Build history of the part. All positions in model axes, mm. A direction names the side the tool comes from. Round coordinates to 2 decimals unless told otherwise and drop trailing zeros. Order: outer loops, then holes, each group sorted by start corner. A loop starts at its lowest first (then second) coordinate and runs counter-clockwise, first axis right, second up. Notation, with made-up numbers: (-31, 24.5) -> (21, 24.5) arc R32 cw to (21, 55.5) -> close; hole circle Ø11 at (68.25, 44). An arc over 180 degrees is marked (long way). Write item = value, one per line.
from build123d import *

# Parameters (mm, degrees)
BOSS_EXTRU_1_DEPTH      = 704
ENL_V_MAT_EXTRU_1_DEPTH = 590
ENL_V_MAT_EXTRU_2_DEPTH = 590
ENL_V_MAT_EXTRU_3_DEPTH = 41
ENL_V_MAT_EXTRU_4_DEPTH = 41


with BuildPart() as part:
    # Esquisse1 → Boss.-Extru.1 (new body)
    with BuildSketch(Plane(origin=(0, 0, 0), x_dir=(1, 0, 0), z_dir=(0, 1, 0))):
        Polygon((-20, 20.113636364), (20, 20.113636364), (20, 18.113636364), (-18, 18.113636364), (-18, -19.886363636), (-20, -19.886363636), align=None)
    extrude(amount=BOSS_EXTRU_1_DEPTH)

    # Esquisse2 → Enlèv. mat.-Extru.1 (cut)
    with BuildSketch(Plane(origin=(0, 0, -20.113636364), x_dir=(-1, 0, 0), z_dir=(0, 0, -1))):
        Polygon((20, 0), (-20, 40), (-20, 0), align=None)
    extrude(amount=-ENL_V_MAT_EXTRU_1_DEPTH, mode=Mode.SUBTRACT)

    # Esquisse3 → Enlèv. mat.-Extru.2 (cut)
    with BuildSketch(Plane.ZY.offset(20)):
        Polygon((-20.113636364, 0), (19.886363636, 40), (19.886363636, 0), align=None)
    extrude(amount=-ENL_V_MAT_EXTRU_2_DEPTH, mode=Mode.SUBTRACT)

    # Esquisse4 → Enlèv. mat.-Extru.3 (cut, through all)
    with BuildSketch(Plane.ZY.offset(20)):
        Polygon((-20.113636364, 704), (19.886363636, 664), (19.886363636, 704), align=None)
    extrude(amount=-ENL_V_MAT_EXTRU_3_DEPTH, mode=Mode.SUBTRACT)

    # Esquisse5 → Enlèv. mat.-Extru.4 (cut, through all)
    with BuildSketch(Plane(origin=(0, 0, -20.113636364), x_dir=(-1, 0, 0), z_dir=(0, 0, -1))):
        Polygon((20, 704), (-20, 664), (-20, 704), align=None)
    extrude(amount=-ENL_V_MAT_EXTRU_4_DEPTH, mode=Mode.SUBTRACT)


solid = part.part
Q1. Probe probe 1 along Z at (x, y) = (9, 643); probe 2 along X at (y, z) = (557.5, -7.5). List the from-to ranges inside material, lowest first.
Check values:
probe_1 = -20.11 to -18.11
probe_2 = -20 to -18
Q2. Flat gauge pins, fed straight in: pin 1 (19 mm diameter, centred on x = -7.5, y = 232.5, fed in from +Z); pin 2 (1.5 mm diameter, centred on y = 427, z = -10.5, fed in from +X). Where does each tip first touch, or does it go through?
Check values:
pin_1 = -18.11
pin_2 = -18
Q3. Cut at A-A, the plane y = 105. List the corners of the cut face in (x, z), and give its area (3 significant figures).
Check values:
outline = (-20, -20.11) -> (20, -20.11) -> (20, -18.11) -> (-18, -18.11) -> (-18, 19.89) -> (-20, 19.89) -> close
area = 156 mm²
Q4. Which spindle directions (+Z, -Z, +X, -X, +Y, -Y) get a long thin tool onto all of the face, cutting with end or side? Do faces 1 (the face through (1, 347, -18.114)), 2 (the face through (-20, 347, 0)). Say none if no direction does.
Check values:
face_1 = +Z, +X, +Y, -Y
face_2 = +Z, -Z, -X, +Y, -Y
Q5. Cut at B-B, the plane x = 0. List the corners of the cut face in (y, z).
Check values:
outline = (20, -20.11) -> (684, -20.11) -> (684, -18.11) -> (20, -18.11) -> close
Q6. Cut at C-C, the plane z = -10. List the corners of the cut face in (x, y), and give its area (3 significant figures).
Check values:
outline = (-20, 10.11) -> (-18, 10.11) -> (-18, 693.89) -> (-20, 693.89) -> close
area = 1,370 mm²
